from build123d import *

# Parameters (mm, degrees)
PAD_DEPTH       = 9
SKETCH001_W     = 26.1
SKETCH001_H     = 34.4
POCKET_DEPTH    = 3
SKETCH002_R     = 22.22
PAD001_DEPTH    = 3
SKETCH003_R     = 24.44
PAD002_DEPTH    = 3
SKETCH004_R     = 26.6
PAD003_DEPTH    = 3
SKETCH005_R     = 28
PAD004_DEPTH    = 3
SKETCH006_R     = 29
PAD005_DEPTH    = 3
SKETCH007_R     = 29
PAD006_DEPTH    = 3
SKETCH008_R     = 29
PAD007_DEPTH    = 3
SKETCH009_W     = 17
SKETCH009_H     = 24
POCKET001_DEPTH = 3
SKETCH010_W     = 16
SKETCH010_H     = 9
POCKET002_DEPTH = 7


with BuildPart() as part:
    # Sketch → Pad (new body)
    with BuildSketch(Plane.XY):
        Polygon((44, 0), (22, 38.105118), (-22, 38.105118), (-44, 0), (-22, -38.105118), (22, -38.105118), align=None)
    extrude(amount=PAD_DEPTH)

    # Sketch001 (on Face8 of Pad) → Pocket (cut)
    with BuildSketch(Plane.XY.offset(9)):
        with Locations((0, -13.905118)):
            Rectangle(SKETCH001_W, SKETCH001_H)
    extrude(amount=-POCKET_DEPTH, mode=Mode.SUBTRACT)

    # Sketch002 (on Face5 of Pocket) → Pad001 (join)
    with BuildSketch(Plane.XY.offset(9)):
        Polygon((22, 38.105118), (-22, 38.105118), (-44, 0), (-22, -38.105118), (22, -38.105118), (44, 0), align=None)
        Circle(SKETCH002_R, mode=Mode.SUBTRACT)
    extrude(amount=PAD001_DEPTH)

    # Sketch003 (on Face14 of Pad001) → Pad002 (join)
    with BuildSketch(Plane.XY.offset(12)):
        Polygon((40, 0), (20, 34.641016), (-20, 34.641016), (-40, 0), (-20, -34.641016), (20, -34.641016), align=None)
        Circle(SKETCH003_R, mode=Mode.SUBTRACT)
    extrude(amount=PAD002_DEPTH)

    # Sketch004 (on Face21 of Pad002) → Pad003 (join)
    with BuildSketch(Plane.XY.offset(15)):
        Polygon((41, 0), (20.5, 35.507042), (-20.5, 35.507042), (-41, 0), (-20.5, -35.507042), (20.5, -35.507042), align=None)
        Circle(SKETCH004_R, mode=Mode.SUBTRACT)
    extrude(amount=PAD003_DEPTH)

    # Sketch005 (on Face28 of Pad003) → Pad004 (join)
    with BuildSketch(Plane.XY.offset(18)):
        Polygon((19, 32.908965), (-19, 32.908965), (-38, 0), (-19, -32.908965), (19, -32.908965), (38, 0), align=None)
        Circle(SKETCH005_R, mode=Mode.SUBTRACT)
    extrude(amount=PAD004_DEPTH)

    # Sketch006 (on Face35 of Pad004) → Pad005 (join)
    with BuildSketch(Plane.XY.offset(21)):
        Polygon((39, 0), (19.5, 33.774991), (-19.5, 33.774991), (-39, 0), (-19.5, -33.774991), (19.5, -33.774991), align=None)
        Circle(SKETCH006_R, mode=Mode.SUBTRACT)
    extrude(amount=PAD005_DEPTH)

    # Sketch007 (on Face42 of Pad005) → Pad006 (join)
    with BuildSketch(Plane.XY.offset(24)):
        Polygon((36, 0), (18, 31.176915), (-18, 31.176915), (-36, 0), (-18, -31.176915), (18, -31.176915), align=None)
        Circle(SKETCH007_R, mode=Mode.SUBTRACT)
    extrude(amount=PAD006_DEPTH)

    # Sketch008 (on Face49 of Pad006) → Pad007 (join)
    with BuildSketch(Plane.XY.offset(27)):
        Polygon((37, 0), (18.5, 32.04294), (-18.5, 32.04294), (-37, 0), (-18.5, -32.04294), (18.5, -32.04294), align=None)
        Circle(SKETCH008_R, mode=Mode.SUBTRACT)
    extrude(amount=PAD007_DEPTH)

    # Sketch009 (on Face74 of Pad007) → Pocket001 (cut)
    with BuildSketch(Plane.XY.offset(6)):
        with Locations((0, -8.705118)):
            Rectangle(SKETCH009_W, SKETCH009_H)
    extrude(amount=-POCKET001_DEPTH, mode=Mode.SUBTRACT)

    # Sketch010 (on Face12 of Pocket001) → Pocket002 (cut)
    with BuildSketch(Plane.XZ.offset(38.105118)):
        with Locations((0, 7.5)):
            Rectangle(SKETCH010_W, SKETCH010_H)
    extrude(amount=-POCKET002_DEPTH, mode=Mode.SUBTRACT)


solid = part.part
Source: CAD feature listing. Evaluate the final solid. Frame: model axes, mm. A direction names the side the tool comes from. Coordinates: 2 decimals unless noted, no trailing zeros. Order: outer loops, then holes, each group sorted by start corner. A loop starts at its lowest first (then second) coordinate and runs counter-clockwise, first axis right, second up.
Item 1: Material intervals for line 1 (Y direction, x = 11.5, z = 24.25); line 2 (Z direction, x = 28, y = 21); line 3 (X direction, y = 0, z = 9.75), sorted ascending.
Output values:
line 1: y = -31.18 to -26.62, 26.62 to 31.18
line 2: z = 0 to 12, 15 to 18
line 3: x = -44 to -22.22, 22.22 to 44
Item 2: Pull-direction query (Z, two-part tool) for faces 5 (the face through (-27.62, 16.25, 28.48)), 6 (the face through (-13.05, -14, 8)), 7 (the face through (25, -10, 18)); classes: pulls with the +Z half, pulls with the -Z half, needs draft (parallel to the pull), parting line crosses it, or undercut.
Output values:
face 5: needs draft
face 6: undercut
face 7: pulls with the +Z half
Item 3: First-contact query: P1, Ø4, axis at x = 14, y = -22, coming from the +Z side; P2, Ø3.5, axis at x = 7, z = 29, coming from the +Y side; P3, Ø1, axis at y = -17, z = 16.5, coming from the -X side. Flat tips, straight axial feed; report the tip coordinate or a pass-through.
Output values:
P1: stops at z = 21
P2: stops at y = 32.04
P3: stops at x = -31.47
Item 4: Cut plane B-B (z = 5). Return loops of the section in (x, y), plus the area to 3 significant figures.
Output values:
outline: (-44, 0) - (-22, -38.11) - (-8, -38.11) - (-8, -31.11) - (8, -31.11) - (8, -38.11) - (22, -38.11) - (44, 0) - (22, 38.11) - (-22, 38.11) - close; hole (-8.5, -20.71) - (8.5, -20.71) - (8.5, 3.29) - (-8.5, 3.29) - close
area: 4,510 mm2
Item 5: Set-up query: faces 1 (the face through (0, 32.909, 19)), 2 (the face through (10, -31.105, 8)), 3 (the face through (12, -22, 15)), 4 (the face through (26.87, -15.81, 25.48)). Return all of +Z, -Z, +X, -X, +Y, -Y with unobstructed straight access to the full face (end or side cutting, diameter ignored); none if empty.
Output values:
face 1: +X, -X, +Y
face 2: none
face 3: +Z
face 4: +X, -Y
Item 6: Cut plane A-A (z = 22). Return loops of the section in (x, y) (3 decimals), plus the area to 3 significant figures.
Output values:
outline: (-39, 0) - (-19.5, -33.775) - (19.5, -33.775) - (39, 0) - (19.5, 33.775) - (-19.5, 33.775) - close; hole circle Ø58 at (0, 0)
area: 1,310 mm2
